```python
from build123d import *

# Parameters (mm, degrees)
BOSS_EXTRUDE1_DEPTH = 21
BOSS_EXTRUDE2_DEPTH = 4
CUT_EXTRUDE1_DEPTH  = 111.552889986
CUT_EXTRUDE2_REACH  = 72.51
FILLET1_R           = 3


with BuildPart() as part:
    # Sketch1 → Boss-Extrude1 (new, symmetric)
    with BuildSketch(Plane(origin=(0, 0, 0), x_dir=(0, 0, -1), z_dir=(1, 0, 0))):
        Polygon((0, 0), (0, 22.987298969), (-46.752018394, 52.201202404), (-60, 31), (-60, 10), (-100, 10), (-100, 0), align=None)
    extrude(amount=BOSS_EXTRUDE1_DEPTH, both=True)

    # Sketch2 → Boss-Extrude2 (add)
    with BuildSketch(Plane(origin=(0, 10, 0), x_dir=(1, 0, 0), z_dir=(0, 1, 0))):
        with BuildLine():
            Line((-9.5, -90), (9.5, -90))
            ThreePointArc((9.5, -90), (16.5, -83), (9.5, -76))
            Line((9.5, -76), (-9.5, -76))
            ThreePointArc((-9.5, -76), (-16.5, -83), (-9.5, -90))
        make_face()
        with BuildLine():
            ThreePointArc((-9.5, -78), (-14.5, -83), (-9.5, -88))
            Line((-9.5, -88), (9.5, -88))
            ThreePointArc((9.5, -88), (14.5, -83), (9.5, -78))
            Line((9.5, -78), (-9.5, -78))
        make_face(mode=Mode.SUBTRACT)
    extrude(amount=BOSS_EXTRUDE2_DEPTH)

    # Sketch2<3> → Cut-Extrude1 (cut, through all)
    with BuildSketch(Plane(origin=(0, 10, 0), x_dir=(1, 0, 0), z_dir=(0, 1, 0))):
        with BuildLine():
            Line((9.5, -78), (-9.5, -78))
            ThreePointArc((-9.5, -78), (-14.5, -83), (-9.5, -88))
            Line((-9.5, -88), (9.5, -88))
            ThreePointArc((9.5, -88), (14.5, -83), (9.5, -78))
        make_face()
    extrude(amount=-CUT_EXTRUDE1_DEPTH, mode=Mode.SUBTRACT)

    # Cut-Extrude2: up to this plane
    cut_extrude2_end = Plane(origin=(21, 0, 0), z_dir=(0, 0, 1))
    # Sketch3 → Cut-Extrude2 (cut, up to the surface)
    with BuildSketch(Plane(origin=(0, 35.669068614, 57.082442121), x_dir=(1, 0, 0), z_dir=(0, 0.5299192642332053, 0.8480480961564258)), mode=Mode.PRIVATE) as cut_extrude2_sk1:
        Polygon((0, 19.494335127), (0, 12.494335127), (11.5, 12.494335127), (6.598547233, 19.494335127), align=None)
    cut_extrude2_tool1 = split(extrude(cut_extrude2_sk1.sketch, amount=-CUT_EXTRUDE2_REACH, mode=Mode.PRIVATE), bisect_by=cut_extrude2_end, keep=Keep.BOTH, mode=Mode.PRIVATE)
    add(cut_extrude2_tool1.solids().sort_by_distance((4.635255, 48.965087, 48.774167))[0], mode=Mode.SUBTRACT)
    # Sketch3 → Cut-Extrude2 (cut, up to the surface)
    with BuildSketch(Plane(origin=(0, 35.669068614, 57.082442121), x_dir=(1, 0, 0), z_dir=(0, 0.5299192642332053, 0.8480480961564258)), mode=Mode.PRIVATE) as cut_extrude2_sk2:
        Polygon((0, 19.494335127), (-6.598547233, 19.494335127), (-11.5, 12.494335127), (0, 12.494335127), align=None)
    cut_extrude2_tool2 = split(extrude(cut_extrude2_sk2.sketch, amount=-CUT_EXTRUDE2_REACH, mode=Mode.PRIVATE), bisect_by=cut_extrude2_end, keep=Keep.BOTH, mode=Mode.PRIVATE)
    add(cut_extrude2_tool2.solids().sort_by_distance((-4.635255, 48.965087, 48.774167))[0], mode=Mode.SUBTRACT)

    # Fillet1
    fillet1_edges = [part.edges().sort_by_distance(p)[0] for p in [
        (21, 5, 100),
        (-21, 5, 100),
        (21, 11.493649485, 0),
        (-21, 11.493649485, 0),
    ]]
    fillet(fillet1_edges, radius=FILLET1_R)


solid = part.part
```
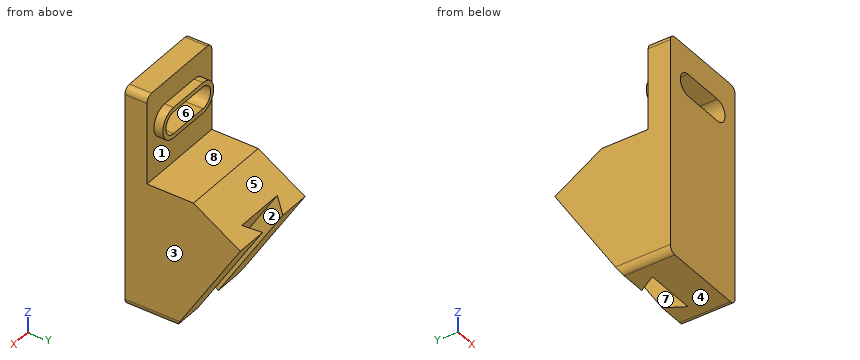
Geometry: final body of the model. Coordinates: model frame, mm. Face numbers are marked on the shaded views. A direction names the side the tool comes from. Round coordinates to 2 decimals unless told otherwise and drop trailing zeros. Loops run counter-clockwise (first coordinate to the right, second up) from the corner with the lowest first, then second, coordinate; pieces in that order, holes last.
Item 1: Section D-D, the plane y = 26. Output: boundary loops of the cut face in (x, z).
Checked values:
outline: (-21, 4.82) - (-6.6, 4.82) - (-11.5, 18.03) - (11.5, 18.03) - (6.6, 4.82) - (21, 4.82) - (21, 60) - (-21, 60) - close
Item 2: Line query: L1, parallel to Z at x = -6.5, y = 12.5; L2, parallel to Y at x = -12, z = 74; L3, parallel to X at y = 28, z = 10. Output: solid intervals per line, ascending.
Checked values:
L1: z = 0 to 60, 76 to 78, 88 to 90
L2: y = 0 to 10
L3: x = -21 to -7.33, 7.33 to 21
Item 3: Section C-C, the plane z = 42. Output: boundary loops of the cut face in (x, y).
Checked values:
outline: (-21, 0) - (21, 0) - (21, 49.23) - (6.6, 49.23) - (11.5, 40.98) - (-11.5, 40.98) - (-6.6, 49.23) - (-21, 49.23) - close
Item 4: Section A-A, the plane y = 13. Output: boundary loops of the cut face in (x, z).
Checked values:
outline: (-21, 3) arc R3 ccw to (-18, 0) - (18, 0) arc R3 ccw to (21, 3) - (21, 60) - (-21, 60) - close; (-9.5, 76) - (9.5, 76) arc R7 ccw to (9.5, 90) - (-9.5, 90) arc R7 ccw to start; hole (-9.5, 78) - (9.5, 78) arc R5 ccw to (9.5, 88) - (-9.5, 88) arc R5 ccw to start
Item 5: Section B-B, the plane z = 83. Output: boundary loops of the cut face in (x, y), plus the area to 3 significant figures.
Checked values:
outline: (-21, 0) - (-14.5, 0) - (-14.5, 14) - (-16.5, 14) - (-16.5, 10) - (-21, 10) - close; (14.5, 0) - (21, 0) - (21, 10) - (16.5, 10) - (16.5, 14) - (14.5, 14) - close
area: 146 mm2
Item 6: Reachability of the marked faces 4, 5, 6, 7 and 8 from +Z, -Z, +X, -X, +Y, -Y: full face, straight path, thin tool, end or side. Return the list, or none.
Checked values:
face 4: -Z, +X, -X, +Y, -Y
face 5: +Z, +X, -X, +Y
face 6: +Y, -Y
face 7: none
face 8: +X, -X, +Y
Item 7: Mould query, pull axis Y, two halves, no side actions, for the marked faces 1, 2 and 3. Classes: released by +Y, released by -Y, zero draft, split by the parting line, or undercut.
Checked values:
face 1: released by +Y
face 2: undercut
face 3: zero draft
Item 8: Contact query for flat-ended pins moving along their axis: P1, Ø6.5, axis at x = 1, y = 23.5, coming from the +Z side; P2, Ø3, axis at x = -8.5, y = 44, coming from the +Z side; P3, Ø12, axis at x = 3.5, y = 17, coming from the +Z side. Output: stop coordinate, or through.
Checked values:
P1: stops at z = 60
P2: stops at z = 52.81
P3: stops at z = 90
